from build123d import *

# Parameters (mm, degrees)
ESQUISSE1_W      = 8
ESQUISSE1_H      = 3
EXTRUSION1_DEPTH = 4
ESQUISSE2_W      = 8
ESQUISSE2_H      = 4
EXTRUSION2_DEPTH = 4.5
ESQUISSE3_R      = 0.75
EXTRUSION3_DEPTH = 10


with BuildPart() as part:
    # Esquisse1 → Extrusion1 (new body)
    with BuildSketch(Plane(origin=(0, 0, 0), x_dir=(1, 0, 0), z_dir=(0, 1, 0))):
        with Locations((4, -1.5)):
            Rectangle(ESQUISSE1_W, ESQUISSE1_H)
    extrude(amount=EXTRUSION1_DEPTH)

    # Esquisse2 → Extrusion2 (add)
    with BuildSketch(Plane(origin=(0, 4, 0), x_dir=(1, 0, 0), z_dir=(0, 1, 0))):
        with Locations((4, -2)):
            Rectangle(ESQUISSE2_W, ESQUISSE2_H)
    extrude(amount=EXTRUSION2_DEPTH)

    # Esquisse3 → Extrusion3 (add)
    with BuildSketch(Plane(origin=(0, 8.5, 0), x_dir=(1, 0, 0), z_dir=(0, 1, 0))):
        with Locations((4, -2)):
            Circle(ESQUISSE3_R)
        with Locations((2, -2)):
            Circle(ESQUISSE3_R)
        with Locations((6, -2)):
            Circle(ESQUISSE3_R)
    extrude(amount=EXTRUSION3_DEPTH)


solid = part.part
Could you check a few things on this model? Use its own coordinates, in mm. A direction names the side the tool comes from. Give positions to 0.01 mm unless a question says otherwise; leave off trailing zeros. Order: outer loops, then holes, each group sorted by start corner. A loop starts at its lowest first (then second) coordinate and runs counter-clockwise, first axis right, second up. Notation, with made-up numbers: (44.25, 14) -> (83.25, 14) arc R30 cw to (83.25, 40) -> close; hole circle Ø5 at (-20.5, 30.25). An arc over 180 degrees is marked (long way). Answer in a Markdown table with one row per item. Add a question column.
Item 1: We'd pull the mould along X, two halves only. Please class faces 4 (the flat face through (8, 4, 2)), 5 (the cylindrical face through (3.45, 13.43, 1.49)), 6 (the cylindrical face through (5.45, 13.43, 1.49)), 7 (the flat face through (3.9, 4, 3.5)): pulls with the +X half, pulls with the -X half, needs draft (parallel to the pull), parting line crosses it, or undercut.
Item 2: Imagine slicing it at D-D (x = 3). List the corners of the cut face in (y, z) for me, and give its area (3 significant figures).
Item 3: For faces 1 (the flat face through (4, 2, 3)), 2 (the flat face through (4, 4, 0)), 3 (the flat face through (3, 8.5, 2)), which set-ups out of +Z, -Z, +X, -X, +Y, -Y let a thin tool reach every point of the face, with its end or its side?
Item 4: I'm going to push flat-ended pins straight in: P1, Ø2, axis at x = 2.5, y = 2.5, coming from the +Z side; P2, Ø0.5, axis at x = 5.5, z = 3.5, coming from the -Y side. Where does each tip first touch, or does it pass through?
Item 5: Imagine slicing it at A-A (x = 4). List the corners of the cut face in (y, z) for me, and give its area (3 significant figures).
Item 6: Imagine slicing it at C-C (z = 2). List the corners of the cut face in (x, y) for me.
Item 7: Imagine slicing it at B-B (y = 16.5). List the corners of the cut face in (x, z) for me.
Item 8: Please list where these lines run through material, in increasing order: probe 1 along X at (y, z) = (9, 2.15); probe 2 along X at (y, z) = (10, 1.35); probe 3 along Y at (x, z) = (1, 3.7).
Result:
| question | item | result |
|---|---|---|
| 1 | face 4 | pulls with the +X half |
| 1 | face 5 | undercut |
| 1 | face 6 | undercut |
| 1 | face 7 | needs draft |
| 2 | outline | (0, 0) -> (8.5, 0) -> (8.5, 4) -> (4, 4) -> (4, 3) -> (0, 3) -> close |
| 2 | area | 30.0 mm2 |
| 3 | face 1 | +Z, +X, -X, -Y |
| 3 | face 2 | -Z, +X, -X, +Y, -Y |
| 3 | face 3 | +Y |
| 4 | P1 | z = 3 |
| 4 | P2 | y = 4 |
| 5 | outline | (0, 0) -> (8.5, 0) -> (8.5, 1.25) -> (18.5, 1.25) -> (18.5, 2.75) -> (8.5, 2.75) -> (8.5, 4) -> (4, 4) -> (4, 3) -> (0, 3) -> close |
| 5 | area | 45.0 mm2 |
| 6 | outline | (0, 0) -> (8, 0) -> (8, 8.5) -> (6.75, 8.5) -> (6.75, 18.5) -> (5.25, 18.5) -> (5.25, 8.5) -> (4.75, 8.5) -> (4.75, 18.5) -> (3.25, 18.5) -> (3.25, 8.5) -> (2.75, 8.5) -> (2.75, 18.5) -> (1.25, 18.5) -> (1.25, 8.5) -> (0, 8.5) -> close |
| 7 | outline | circle Ø1.5 at (2, 2); circle Ø1.5 at (4, 2); circle Ø1.5 at (6, 2) |
| 8 | probe 1 | 1.27 to 2.73, 3.27 to 4.73, 5.27 to 6.73 |
| 8 | probe 2 | 1.63 to 2.37, 3.63 to 4.37, 5.63 to 6.37 |
| 8 | probe 3 | 4 to 8.5 |
